Input: part model. Units: mm. Frame: model coordinates. Face numbers are marked on the shaded views. A direction names the side the tool comes from. Round coordinates to 2 decimals unless told otherwise and drop trailing zeros. Loops run counter-clockwise (first coordinate to the right, second up) from the corner with the lowest first, then second, coordinate; pieces in that order, holes last. Notation, with made-up numbers: (43.5, -28.5) -> (92.5, -28.5) arc R24 cw to (92.5, -10.5) -> close; hole circle Ø11 at (-24, 69). An arc over 180 degrees is marked (long way). Answer as a JSON object with one key per item and string values. Group by question number.
Item 1: Material intervals for line 1 (X direction, y = 97, z = 96); line 2 (Z direction, x = 374, y = 102.5); line 3 (Y direction, x = 172, z = 84), sorted ascending. Write a range as [from, to].
Item 2: Pin query (flat end, axial travel): pin 1 (6 mm diameter, centred on x = -80.5, z = -1.5, fed in from +Y). Return the tip coordinate at first contact, or that it passes through.
Item 3: Draft query along X for the marked faces 1, 2 and 3. Return one class per face: released by +X, released by -X, zero draft, split by the parting line, or undercut.
Item 4: Section query B-B on y = 61. Return loops of the section in (x, z).
Item 5: Section query A-A on z = -63.75. Return loops of the section in (x, y).
Item 6: Set-up query: the marked faces 4 and 5. Return all of +Z, -Z, +X, -X, +Y, -Y with unobstructed straight access to the full face (end or side cutting, diameter ignored); none if empty.
Item 7: Section query C-C on x = 221. Return loops of the section in (y, z).
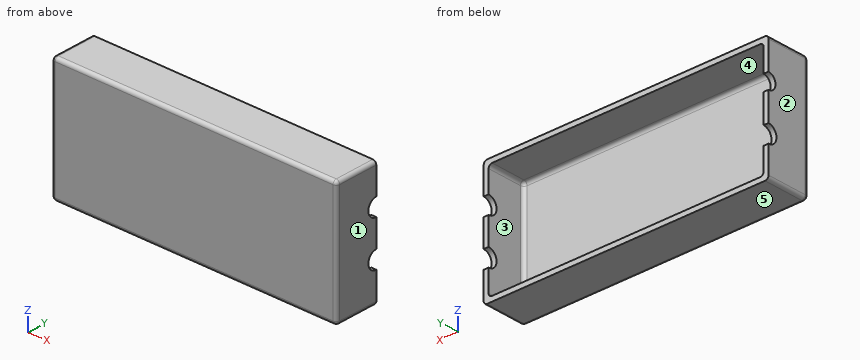
from build123d import *

# Parameters (mm, degrees)
SKETCH1_W           = 814
SKETCH1_H           = 350
BOSS_EXTRUDE1_DEPTH = 125
SKETCH2_W           = 786
SKETCH2_H           = 322
CUT_EXTRUDE1_DEPTH  = 110
FILLET1_R           = 10
FILLET2_R           = 10
FILLET3_R           = 10
SKETCH4_R           = 25
SKETCH4_R_2         = 22
CUT_EXTRUDE2_DEPTH  = 110
CUT_EXTRUDE3_START  = -110
SKETCH5_R           = 25
CUT_EXTRUDE3_DEPTH  = 110


with BuildPart() as part:
    # Sketch1 → Boss-Extrude1 (new body)
    with BuildSketch(Plane(origin=(0, 0, 0), x_dir=(1, 0, 0), z_dir=(0, 1, 0))):
        Rectangle(SKETCH1_W, SKETCH1_H)
    extrude(amount=BOSS_EXTRUDE1_DEPTH)

    # Sketch2 → Cut-Extrude1 (cut)
    with BuildSketch(Plane(origin=(0, 125, 0), x_dir=(1, 0, 0), z_dir=(0, 1, 0))):
        Rectangle(SKETCH2_W, SKETCH2_H)
    extrude(amount=-CUT_EXTRUDE1_DEPTH, mode=Mode.SUBTRACT)

    # Fillet1
    fillet1_edges = [part.edges().sort_by_distance(p)[0] for p in [
        (0, 0, -175),
        (407, 0, 0),
        (0, 0, 175),
        (-407, 0, 0),
    ]]
    fillet(fillet1_edges, radius=FILLET1_R)

    # Fillet2
    # the kernel refuses this fillet: 10 mm, written as the material it takes off along each edge
    with BuildSketch(Plane(origin=(397, 10, -165), x_dir=(0, 0, -1), z_dir=(1, 0, 0))) as fillet2_piece_1_section:
        Polygon((0, 0), (FILLET2_R, 0), (FILLET2_R, -FILLET2_R), (0, -FILLET2_R), align=None)
    fillet2_piece_1 = extrude(amount=FILLET2_R, mode=Mode.PRIVATE)
    fillet2_piece_1 = fillet2_piece_1 - Plane(origin=(397, 10, -165), x_dir=(0, 0.7071067811865475, 0.7071067811865475), z_dir=(1, 0, 0)) * Sphere(FILLET2_R, mode=Mode.PRIVATE)
    add(fillet2_piece_1, mode=Mode.SUBTRACT)
    with BuildSketch(Plane(origin=(397, 10, 165), x_dir=(1, 0, 0), z_dir=(0, 0, 1))) as fillet2_piece_2_section:
        Polygon((0, 0), (FILLET2_R, 0), (FILLET2_R, -FILLET2_R), (0, -FILLET2_R), align=None)
    fillet2_piece_2 = extrude(amount=FILLET2_R, mode=Mode.PRIVATE)
    fillet2_piece_2 = fillet2_piece_2 - Plane(origin=(397, 10, 165), x_dir=(-0.7071067811865475, 0.7071067811865475, 0), z_dir=(0, 0, 1)) * Sphere(FILLET2_R, mode=Mode.PRIVATE)
    add(fillet2_piece_2, mode=Mode.SUBTRACT)
    with BuildSketch(Plane(origin=(-397, 10, -165), x_dir=(0, 0, -1), z_dir=(-1, 0, 0))) as fillet2_piece_3_section:
        Polygon((0, 0), (FILLET2_R, 0), (FILLET2_R, FILLET2_R), (0, FILLET2_R), align=None)
    fillet2_piece_3 = extrude(amount=FILLET2_R, mode=Mode.PRIVATE)
    fillet2_piece_3 = fillet2_piece_3 - Plane(origin=(-397, 10, -165), x_dir=(0, 0.7071067811865475, 0.7071067811865475), z_dir=(-1, 0, 0)) * Sphere(FILLET2_R, mode=Mode.PRIVATE)
    add(fillet2_piece_3, mode=Mode.SUBTRACT)
    with BuildSketch(Plane(origin=(-397, 10, 165), x_dir=(-1, 0, 0), z_dir=(0, 0, 1))) as fillet2_piece_4_section:
        Polygon((0, 0), (FILLET2_R, 0), (FILLET2_R, FILLET2_R), (0, FILLET2_R), align=None)
    fillet2_piece_4 = extrude(amount=FILLET2_R, mode=Mode.PRIVATE)
    fillet2_piece_4 = fillet2_piece_4 - Plane(origin=(-397, 10, 165), x_dir=(0.7071067811865475, 0.7071067811865475, 0), z_dir=(0, 0, 1)) * Sphere(FILLET2_R, mode=Mode.PRIVATE)
    add(fillet2_piece_4, mode=Mode.SUBTRACT)
    with BuildSketch(Plane(origin=(-407, 10, -175), x_dir=(0, 0, 1), z_dir=(0, 1, 0)), Plane(origin=(-407, 10, 175), x_dir=(1, 0, 0), z_dir=(0, 1, 0))) as fillet2_piece_5:
        with BuildLine():
            CenterArc((FILLET2_R, FILLET2_R), FILLET2_R, 180, 90)
            Line((0, FILLET2_R), (0, 0))
            Line((0, 0), (FILLET2_R, 0))
        make_face()
    extrude(amount=140, mode=Mode.SUBTRACT)
    with BuildSketch(Plane(origin=(407, 10, -175), x_dir=(0, 0, 1), z_dir=(0, 1, 0)), Plane(origin=(407, 10, 175), x_dir=(-1, 0, 0), z_dir=(0, 1, 0))) as fillet2_piece_6:
        with BuildLine():
            CenterArc((FILLET2_R, -FILLET2_R), FILLET2_R, 90, 90)
            Line((0, -FILLET2_R), (0, 0))
            Line((0, 0), (FILLET2_R, 0))
        make_face()
    extrude(amount=140, mode=Mode.SUBTRACT)

    # Fillet3
    fillet3_edges = [part.edges().sort_by_distance(p)[0] for p in [
        (393, 15, 0),
        (393, 70, -161),
        (0, 15, 161),
        (393, 70, 161),
        (-393, 15, 0),
        (-393, 70, 161),
        (0, 15, -161),
        (-393, 70, -161),
    ]]
    fillet(fillet3_edges, radius=FILLET3_R)

    # Sketch4 → Cut-Extrude2 (cut)
    with BuildSketch(Plane.ZY.offset(407)):
        with Locations((-63.75, 125)):
            Circle(SKETCH4_R)
        with Locations((63.75, 125)):
            Circle(SKETCH4_R_2)
    extrude(amount=-CUT_EXTRUDE2_DEPTH, mode=Mode.SUBTRACT)

    # Sketch5 → Cut-Extrude3 (cut)
    with BuildSketch(Plane(origin=(407, 0, 0), x_dir=(0, 0, -1), z_dir=(1, 0, 0)).offset(CUT_EXTRUDE3_START)):
        with Locations((-63.75, 125)):
            Circle(SKETCH5_R)
        with Locations((63.75, 125)):
            Circle(SKETCH5_R)
    extrude(amount=CUT_EXTRUDE3_DEPTH, mode=Mode.SUBTRACT)


solid = part.part
Solved:
{
 "1": {"line 1": "[-407, -393], [393, 407]", "line 2": "[-175, -161], [161, 175]", "line 3": "[0, 15]"},
 "2": {"pin 1": "y = 15"},
 "3": {"face 1": "released by +X", "face 2": "released by -X", "face 3": "undercut"},
 "4": {"outline": "(-407, -165) arc R10 ccw to (-397, -175) -> (397, -175) arc R10 ccw to (407, -165) -> (407, 165) arc R10 ccw to (397, 175) -> (-397, 175) arc R10 ccw to (-407, 165) -> close; hole (-393, -151) arc R10 ccw to (-383, -161) -> (383, -161) arc R10 ccw to (393, -151) -> (393, 151) arc R10 ccw to (383, 161) -> (-383, 161) arc R10 ccw to (-393, 151) -> close"},
 "5": {"outline": "(-407, 10) arc R10 ccw to (-397, 0) -> (397, 0) arc R10 ccw to (407, 10) -> (407, 100) -> (393, 100) -> (393, 25) arc R10 cw to (383, 15) -> (-383, 15) arc R10 cw to (-393, 25) -> (-393, 100) -> (-407, 100) -> close"},
 "6": {"face 4": "+Y", "face 5": "-Z, +X, -X, +Y, -Y"},
 "7": {"outline": "(0, -165) arc R10 ccw to (10, -175) -> (125, -175) -> (125, -161) -> (25, -161) arc R10 cw to (15, -151) -> (15, 151) arc R10 cw to (25, 161) -> (125, 161) -> (125, 175) -> (10, 175) arc R10 ccw to (0, 165) -> close"}
}
